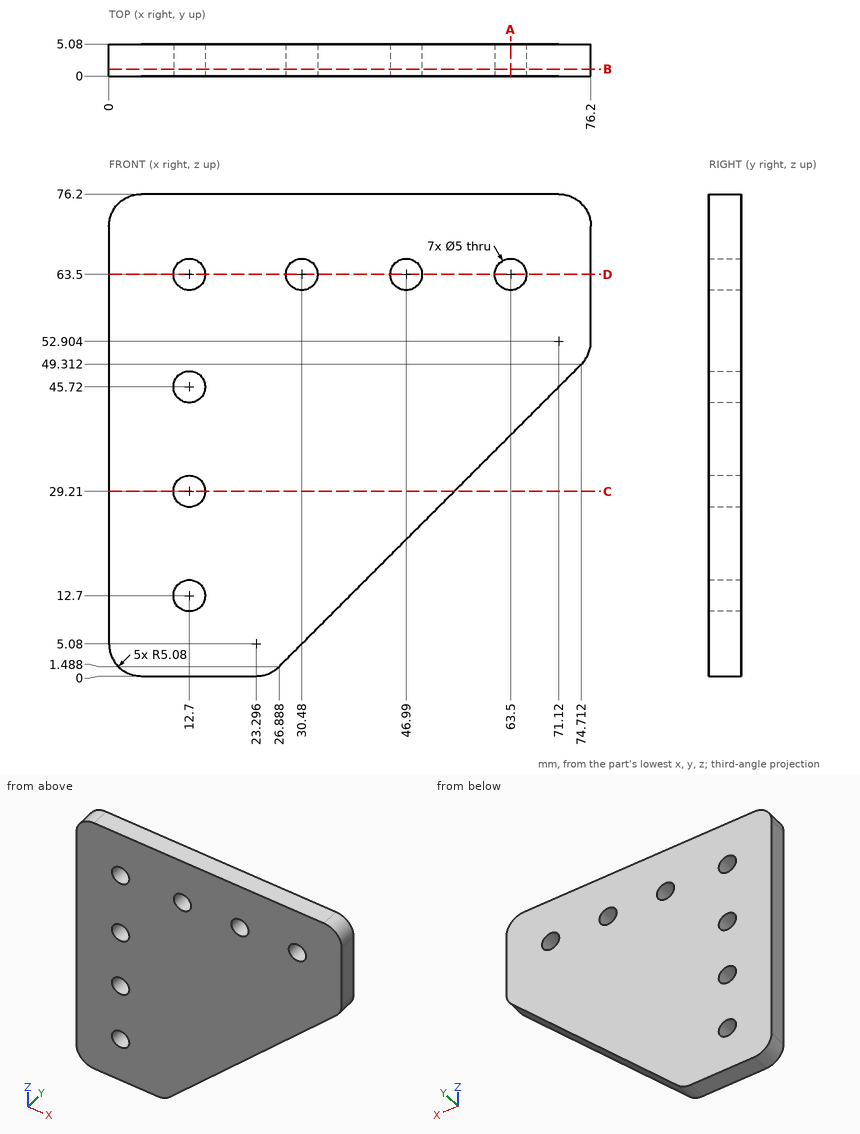
The drawing under review shows one solid part. Ordinate dimensions are in mm from its lowest x, y, z. Round coordinates to 2 decimals unless told otherwise and drop trailing zeros. Loops run counter-clockwise (first coordinate to the right, second up) from the corner with the lowest first, then second, coordinate; pieces in that order, holes last. Notation, with made-up numbers: (-34.5, 46.25) -> (-4.5, 46.25) arc R23 ccw to (-4.5, 63.25) -> close; hole circle Ø9 at (65.25, -2). An arc over 180 degrees is marked (long way). Answer in a Markdown table with one row per item.
1) Consider section A-A, the plane x = 63.5. Write out the cut boundary in (y, z).
Taken from the geometry:
| item | result |
|---|---|
| outline | (0, 38.1) -> (5.08, 38.1) -> (5.08, 61) -> (0, 61) -> close; (0, 66) -> (5.08, 66) -> (5.08, 76.2) -> (0, 76.2) -> close |
2) Consider section C-C, the plane z = 29.21. Write out the cut boundary in (x, y), plus the area to 3 significant figures.
Taken from the geometry:
| item | result |
|---|---|
| outline | (0, 0) -> (10.2, 0) -> (10.2, 5.08) -> (0, 5.08) -> close; (15.2, 0) -> (54.61, 0) -> (54.61, 5.08) -> (15.2, 5.08) -> close |
| area | 252 mm² |
3) For pin 1 Ø4 at (x, z) = (12.7, 29.21) entering from -Y, flat-tipped, find the tip position at first contact; note if it passes through.
Taken from the geometry:
| item | result |
|---|---|
| pin 1 | passes through |
4) Consider section D-D, the plane z = 63.5. Write out the cut boundary in (x, y).
Taken from the geometry:
| item | result |
|---|---|
| outline | (0, 0) -> (10.2, 0) -> (10.2, 5.08) -> (0, 5.08) -> close; (15.2, 0) -> (27.98, 0) -> (27.98, 5.08) -> (15.2, 5.08) -> close; (32.98, 0) -> (44.49, 0) -> (44.49, 5.08) -> (32.98, 5.08) -> close; (49.49, 0) -> (61, 0) -> (61, 5.08) -> (49.49, 5.08) -> close; (66, 0) -> (76.2, 0) -> (76.2, 5.08) -> (66, 5.08) -> close |
5) Consider section B-B, the plane y = 1.1. Write out the cut boundary in (x, z), plus the area to 3 significant figures.
Taken from the geometry:
| item | result |
|---|---|
| outline | (0, 5.08) arc R5.08 ccw to (5.08, 0) -> (23.3, 0) arc R5.08 ccw to (26.89, 1.49) -> (74.71, 49.31) arc R5.08 ccw to (76.2, 52.9) -> (76.2, 71.12) arc R5.08 ccw to (71.12, 76.2) -> (5.08, 76.2) arc R5.08 ccw to (0, 71.12) -> close; hole circle Ø5 at (12.7, 12.7); hole circle Ø5 at (12.7, 29.21); hole circle Ø5 at (12.7, 45.72); hole circle Ø5 at (12.7, 63.5); hole circle Ø5 at (30.48, 63.5); hole circle Ø5 at (46.99, 63.5); hole circle Ø5 at (63.5, 63.5) |
| area | 4,360 mm² |
6) Wall thickness on line 1 along X through (y, z) = (2.75, 63.5); line 2 along Z through (x, y) = (65.5, 3); line 3 along X through (y, z) = (4.9, 13.5): over which ranges is each line inside the solid? List them lowest first.
Taken from the geometry:
| item | result |
|---|---|
| line 1 | x = 0 to 10.2, 15.2 to 27.98, 32.98 to 44.49, 49.49 to 61, 66 to 76.2 |
| line 2 | z = 40.1 to 62, 65 to 76.2 |
| line 3 | x = 0 to 10.33, 15.07 to 38.9 |
